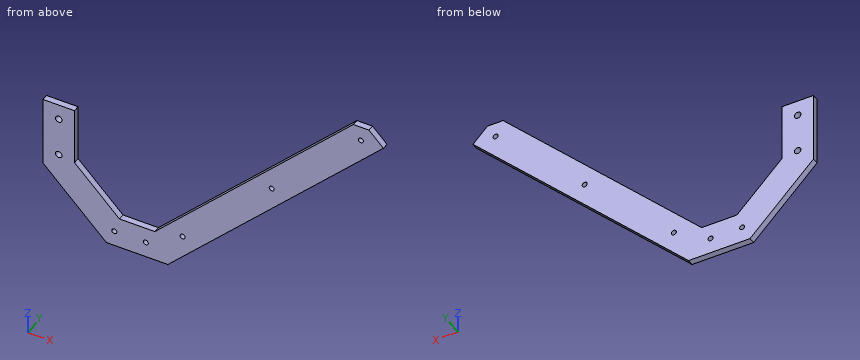
from build123d import *

# Parameters (mm, degrees)
SKETCH_1_R          = 2.1
EXTRUDE_1_DEPTH     = 4
CUT_EXTRUDE_1_DEPTH = 10
SKETCH_3_R          = 1.6
CUT_EXTRUDE_2_DEPTH = 50
CUT_EXTRUDE_3_DEPTH = 50
SKETCH_5_R          = 1.6
CUT_EXTRUDE_4_DEPTH = 50


with BuildPart() as part:
    # 草图1 → 凸台-拉伸1 (new body)
    with BuildSketch(Plane(origin=(0, 0, 0), x_dir=(1, 0, 0), z_dir=(0, 1, 0))):
        Polygon((20, 0), (0, 0), (0, 45), (40.25, 85.25), (79.25, 85.25), (225.25, -60.75), (225.25, -99.75), (185, -140), (140, -140), (140, -120), (176.715728753, -120), (205.25, -91.465728753), (205.25, -69.034271247), (70.965728753, 65.25), (48.534271247, 65.25), (20, 36.715728753), align=None)
        with Locations(Location((10, 10, 0), (0, 0, 270))):
            Circle(SKETCH_1_R, mode=Mode.SUBTRACT)
        with Locations(Location((10, 35, 0), (0, 0, 90))):
            Circle(SKETCH_1_R, mode=Mode.SUBTRACT)
        with Locations(Location((175, -130, 0), (0, 0, 270))):
            Circle(SKETCH_1_R, mode=Mode.SUBTRACT)
        with Locations(Location((150, -130, 0), (0, 0, 90))):
            Circle(SKETCH_1_R, mode=Mode.SUBTRACT)
    extrude(amount=EXTRUDE_1_DEPTH)

    # 草图2 → 切除-拉伸1 (cut)
    with BuildSketch(Plane(origin=(0, 4, 0), x_dir=(1, 0, 0), z_dir=(0, 1, 0))):
        Polygon((225.25, -60.75), (225.25, -99.75), (185, -140), (140, -140), (140, -120), (176.715728753, -120), (205.25, -91.465728753), (205.25, -69.034271247), (196.965728753, -60.75), align=None)
    extrude(amount=-CUT_EXTRUDE_1_DEPTH, mode=Mode.SUBTRACT)

    # 草图3 → 切除-拉伸2 (cut)
    with BuildSketch(Plane(origin=(0, 4, 0), x_dir=(1, 0, 0), z_dir=(0, 1, 0))):
        with Locations(Location((201.747474683, -51.389610307, 0), (0, 0, 270))):
            Circle(SKETCH_3_R)
        with Locations(Location((88.610389693, 61.747474683, 0), (0, 0, 270))):
            Circle(SKETCH_3_R)
        with Locations(Location((145.178932188, 5.178932188, 0), (0, 0, 270))):
            Circle(SKETCH_3_R)
    extrude(amount=-CUT_EXTRUDE_2_DEPTH, mode=Mode.SUBTRACT)

    # 草图4 → 切除-拉伸3 (cut)
    with BuildSketch(Plane(origin=(0, 4, 0), x_dir=(1, 0, 0), z_dir=(0, 1, 0))):
        Polygon((225.25, -60.75), (216.057611845, -51.557611845), (206.865223689, -60.75), align=None)
    extrude(amount=-CUT_EXTRUDE_3_DEPTH, mode=Mode.SUBTRACT)

    # 草图5 → 切除-拉伸4 (cut)
    with BuildSketch(Plane(origin=(0, 4, 0), x_dir=(1, 0, 0), z_dir=(0, 1, 0))):
        with Locations(Location((65.25, 75.25, 0), (0, 0, 270))):
            Circle(SKETCH_5_R)
        with Locations(Location((45.25, 75.25, 0), (0, 0, 270))):
            Circle(SKETCH_5_R)
    extrude(amount=-CUT_EXTRUDE_4_DEPTH, mode=Mode.SUBTRACT)


solid = part.part
Here's how the part is built. I have some questions about the finished solid (model axes, mm). Round coordinates to 2 decimals unless told otherwise and drop trailing zeros. Write each loop counter-clockwise with the first axis right and the second up, starting at its lowest first coordinate (ties: lowest second). Pieces come first, ordered by that corner, then holes.
1. Suppose I cut it at C-C (z = 47). List the corners of the cut face in (x, y) for me.
2. I need wall thicknesses on L1, parallel to X at y = 0.9, z = -35; L2, parallel to X at y = 3.15, z = -10; L3, parallel to Z at x = 65.25, y = 2.35. Which ranges of each line are inside material? Lowest first, please.
3. Suppose I cut it at B-B (y = 2.6). List the corners of the cut face in (x, z) for me, and give its area (3 significant figures).
4. Suppose I cut it at D-D (x = 100). List the corners of the cut face in (y, z) for me.
5. Suppose I cut it at A-A (z = -58). List the corners of the cut face in (x, y) for me.
6. Will these pins go through, and if not, where does the flat tip stop? pin 1 Ø4 at (x, z) = (45.25, -75.25) entering from -Y; pin 2 Ø1.5 at (y, z) = (2.5, -59.5) entering from -X; pin 3 Ø2.5 at (x, z) = (65.25, -75.25) entering from +Y; pin 4 Ø1.5 at (x, y) = (87, 2) entering from +Z.
Answer sheet:
1. outline: (183.22, 0) - (211.5, 0) - (211.5, 4) - (183.22, 4) - close
2. L1: x = 0 to 7.9, 12.1 to 20, 101.22 to 129.5
2. L2: x = 0 to 7.9, 12.1 to 20, 126.22 to 154.5
2. L3: z = -85.25 to -76.85, -73.65 to -65.25
3. outline: (0, -45) - (40.25, -85.25) - (79.25, -85.25) - (216.06, 51.56) - (206.87, 60.75) - (196.97, 60.75) - (70.97, -65.25) - (48.53, -65.25) - (20, -36.72) - (20, 0) - (0, 0) - close; hole circle Ø4.2 at (10, -35); hole circle Ø4.2 at (10, -10); hole circle Ø3.2 at (45.25, -75.25); hole circle Ø3.2 at (65.25, -75.25); hole circle Ø3.2 at (88.61, -61.75); hole circle Ø3.2 at (145.18, -5.18); hole circle Ø3.2 at (201.75, 51.39)
3. area: 6,100 mm2
4. outline: (0, -64.5) - (4, -64.5) - (4, -36.22) - (0, -36.22) - close
5. outline: (13, 0) - (41.28, 0) - (41.28, 4) - (13, 4) - close; (78.22, 0) - (106.5, 0) - (106.5, 4) - (78.22, 4) - close
6. pin 1: stops at y = 0
6. pin 2: stops at x = 13.75
6. pin 3: passes through
6. pin 4: stops at z = -48.47
